Part print with two shaded views. Sizes in mm from the minimum x, y, z corner. Round coordinates to 2 decimals unless told otherwise and drop trailing zeros. Loops run counter-clockwise (first coordinate to the right, second up) from the corner with the lowest first, then second, coordinate; pieces in that order, holes last. Notation, with made-up numbers: (60.25, 44) -> (68.25, 44) arc R13 ccw to (68.25, 61) -> close; hole circle Ø9 at (-6.75, -15). An arc over 180 degrees is marked (long way). Use a Markdown table: item, result. Add a question column.
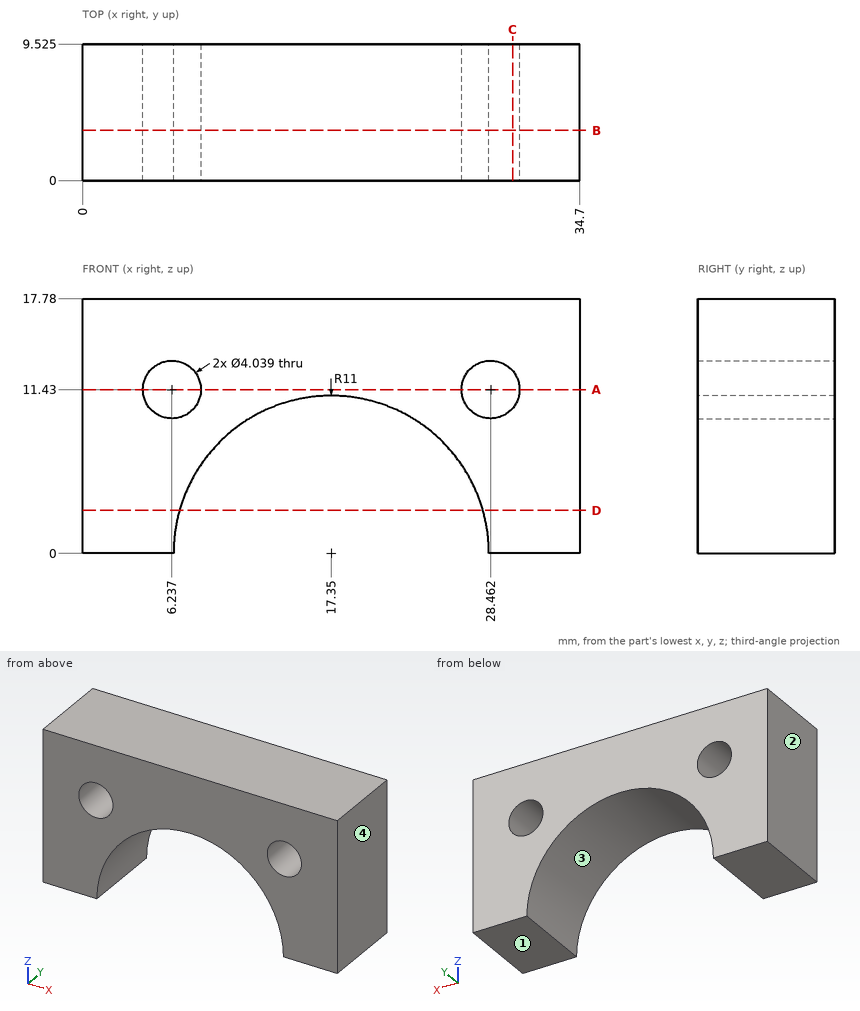
1) Cut at B-B on y = 3.5. Write the cut outline in (x, z).
2) Cut at A-A on z = 11.43. Write the cut outline in (x, y) (1 decimal).
3) Wall check: probe 1 along X at (y, z) = (3, 11.43); probe 2 along X at (y, z) = (7.75, 11.25); probe 3 along X at (y, z) = (2, 10) (1 decimal). Give the ranges that are in metal, low to high. Write a range as from..to.
4) Pull direction X, two halves, no side cores. Call the marked faces 1, 2, 3 and 4: +X half, -X half, draft (parallel to the pull), parting line (faces both ways), or undercut.
5) Cut at C-C on x = 30. Write the cut outline in (y, z) (1 decimal), and give its area (3 significant figures).
6) Cut at D-D on z = 3. Write the cut outline in (x, y) (1 decimal).
Established:
| question | item | result |
|---|---|---|
| 1 | outline | (0, 0) -> (6.35, 0) arc R11 cw to (28.35, 0) -> (34.7, 0) -> (34.7, 17.78) -> (0, 17.78) -> close; hole circle Ø4.04 at (6.24, 11.43); hole circle Ø4.04 at (28.46, 11.43) |
| 2 | outline | (0, 0) -> (4.2, 0) -> (4.2, 9.5) -> (0, 9.5) -> close; (8.3, 0) -> (26.4, 0) -> (26.4, 9.5) -> (8.3, 9.5) -> close; (30.5, 0) -> (34.7, 0) -> (34.7, 9.5) -> (30.5, 9.5) -> close |
| 3 | probe 1 | x = 0..4.22, 8.26..26.44, 30.48..34.7 |
| 3 | probe 2 | x = 0..4.23, 8.25..26.45, 30.47..34.7 |
| 3 | probe 3 | x = 0..4.8, 7.7..12.8, 21.9..27, 29.9..34.7 |
| 4 | face 1 | draft |
| 4 | face 2 | -X half |
| 4 | face 3 | undercut |
| 4 | face 4 | +X half |
| 5 | outline | (0, 0) -> (9.5, 0) -> (9.5, 10.1) -> (0, 10.1) -> close; (0, 12.7) -> (9.5, 12.7) -> (9.5, 17.8) -> (0, 17.8) -> close |
| 5 | area | 144 mm^2 |
| 6 | outline | (0, 0) -> (6.8, 0) -> (6.8, 9.5) -> (0, 9.5) -> close; (27.9, 0) -> (34.7, 0) -> (34.7, 9.5) -> (27.9, 9.5) -> close |
